```python
from build123d import *

# Parameters (mm, degrees)
BOSS_EXTRUDE1_DEPTH = 5
CUT_EXTRUDE1_DEPTH  = 43.772012023
FILLET1_R           = 2.54
SKETCH3_W           = 20
SKETCH3_H           = 10
BOSS_EXTRUDE2_DEPTH = 48
SKETCH4_W           = 16
SKETCH4_H           = 5
CUT_EXTRUDE4_DEPTH  = 32
FILLET2_R           = 2


with BuildPart() as part:
    # Sketch1 → Boss-Extrude1 (new body)
    with BuildSketch(Plane(origin=(0, 0, 0), x_dir=(1, 0, 0), z_dir=(0, 1, 0))):
        Polygon((-29.999623956, -29.926382831), (30.000376044, -29.926382831), (30.000376044, -9.926382831), (10.000376044, -9.926382831), (10.000376044, 10.073617169), (30.000376044, 10.073617169), (30.000376044, 30.073617169), (-29.999623956, 30.073617169), (-29.999623956, 10.073617169), (-9.999623956, 10.073617169), (-9.999623956, -9.926382831), (-29.999623956, -9.926382831), align=None)
    extrude(amount=BOSS_EXTRUDE1_DEPTH)

    # Sketch2 → Cut-Extrude1 (cut, through all)
    with BuildSketch(Plane(origin=(0, 5, 0), x_dir=(1, 0, 0), z_dir=(0, 1, 0))):
        with BuildLine():
            Line((-18.549247911, 18.573617169), (18.55, 18.573617169))
            ThreePointArc((18.55, 18.573617169), (19.575304833, 18.998312337), (20, 20.023617169))
            Line((20, 20.023617169), (20, 20.123617169))
            ThreePointArc((20, 20.123617169), (19.575304833, 21.148922002), (18.55, 21.573617169))
            Line((18.55, 21.573617169), (-18.549247911, 21.573617169))
            ThreePointArc((-18.549247911, 21.573617169), (-19.574552744, 21.148922002), (-19.999247911, 20.123617169))
            Line((-19.999247911, 20.123617169), (-19.999247911, 20.023617169))
            ThreePointArc((-19.999247911, 20.023617169), (-19.574552744, 18.998312337), (-18.549247911, 18.573617169))
        make_face()
        with BuildLine():
            Line((-18.549623956, -21.426382831), (18.550376044, -21.426382831))
            ThreePointArc((18.550376044, -21.426382831), (19.575680877, -21.001687663), (20.000376044, -19.976382831))
            Line((20.000376044, -19.976382831), (20.000376044, -19.876382831))
            ThreePointArc((20.000376044, -19.876382831), (19.575680877, -18.851077998), (18.550376044, -18.426382831))
            Line((18.550376044, -18.426382831), (-18.549623956, -18.426382831))
            ThreePointArc((-18.549623956, -18.426382831), (-19.574928788, -18.851077998), (-19.999623956, -19.876382831))
            Line((-19.999623956, -19.876382831), (-19.999623956, -19.976382831))
            ThreePointArc((-19.999623956, -19.976382831), (-19.574928788, -21.001687663), (-18.549623956, -21.426382831))
        make_face()
    extrude(amount=-CUT_EXTRUDE1_DEPTH, mode=Mode.SUBTRACT)

    # Fillet1
    fillet1_edges = [part.edges().sort_by_distance(p)[0] for p in [
        (-29.999623956, 2.5, -10.073617169),
        (-29.999623956, 2.5, -30.073617169),
        (30.000376044, 2.5, -30.073617169),
        (30.000376044, 2.5, -10.073617169),
        (10.000376044, 2.5, -10.073617169),
        (10.000376044, 2.5, 9.926382831),
        (30.000376044, 2.5, 9.926382831),
        (30.000376044, 2.5, 29.926382831),
        (-29.999623956, 2.5, 29.926382831),
        (-29.999623956, 2.5, 9.926382831),
        (-9.999623956, 2.5, 9.926382831),
        (-9.999623956, 2.5, -10.073617169),
    ]]
    fillet(fillet1_edges, radius=FILLET1_R)

    # Sketch3 → Boss-Extrude2 (add)
    with BuildSketch(Plane(origin=(0, 5, 0), x_dir=(1, 0, 0), z_dir=(0, 1, 0))):
        Rectangle(SKETCH3_W, SKETCH3_H)
    extrude(amount=BOSS_EXTRUDE2_DEPTH)

    # Sketch4 → Cut-Extrude4 (cut)
    with BuildSketch(Plane(origin=(0, 0, -5), x_dir=(-1, 0, 0), z_dir=(0, 0, -1))):
        with Locations((0, 38.5)):
            Rectangle(SKETCH4_W, SKETCH4_H)
    extrude(amount=-CUT_EXTRUDE4_DEPTH, mode=Mode.SUBTRACT)

    # Fillet2
    fillet2_edges = [part.edges().sort_by_distance(p)[0] for p in [
        (0.000188022, 5, 5),
        (0.000188022, 5, -5),
        (10, 53, 0),
        (-10, 53, 0),
        (-8, 41, 0),
        (-8, 36, 0),
        (8, 36, 0),
        (8, 41, 0),
    ]]
    fillet(fillet2_edges, radius=FILLET2_R)


solid = part.part
```
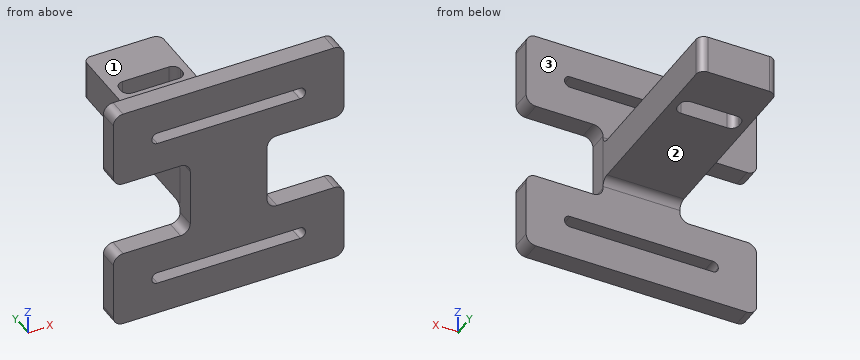
CAD build for the part. Positions are in the model's coordinates, mm. Face numbers are marked on the shaded views. A direction names the side the tool comes from. Round coordinates to 2 decimals unless told otherwise and drop trailing zeros. Order: outer loops, then holes, each group sorted by start corner. A loop starts at its lowest first (then second) coordinate and runs counter-clockwise, first axis right, second up.
Item 1: Saw through at B-B on y = 37. Write the cut outline in (x, z), then the cut area to 3 significant figures.
Item 2: Saw through at A-A on x = -16. Write the cut outline in (y, z), then the cut area to 3 significant figures.
Item 3: Saw through at D-D on x = -22. Write the cut outline in (y, z).
Item 4: Pin check, flat tips, straight feed: pin 1 (3 mm diameter, centred on x = -1, z = -1.5, fed in from -Y); pin 2 (2 mm diameter, centred on x = 8, z = 20.5, fed in from +Y); pin 3 (7 mm diameter, centred on y = 38.5, z = -1.5, fed in from +X); pin 4 (6 mm diameter, centred on x = 3.5, y = 22, fed in from -Z). Stop position of each tip, or through.
Item 5: Probe line 1 along Y through (x, z) = (2, 0); line 2 along Z through (x, y) = (-7.5, 15.5); line 3 along Y through (x, z) = (26, 24). List the from-to ranges inside material, lowest first.
Item 6: Tool access for the marked faces 1, 2 and 3: list every direction of +Z, -Z, +X, -X, +Y, -Y with a clear straight run to the whole face (end or side of a thin tool).
Reported:
1. outline: (-10, -5) - (-7.73, -5) - (-7.73, 5) - (-10, 5) - close; (7.73, -5) - (10, -5) - (10, 5) - (7.73, 5) - close
1. area: 45.4 mm2
2. outline: (0, -30.07) - (5, -30.07) - (5, -21.57) - (0, -21.57) - close; (0, -18.57) - (5, -18.57) - (5, -10.07) - (0, -10.07) - close; (0, 9.93) - (5, 9.93) - (5, 18.43) - (0, 18.43) - close; (0, 21.43) - (5, 21.43) - (5, 29.93) - (0, 29.93) - close
2. area: 170 mm2
3. outline: (0, -30.07) - (5, -30.07) - (5, -10.07) - (0, -10.07) - close; (0, 9.93) - (5, 9.93) - (5, 29.93) - (0, 29.93) - close
4. pin 1: stops at y = 0
4. pin 2: stops at y = 5
4. pin 3: stops at x = 10
4. pin 4: stops at z = -5
5. line 1: y = 0 to 36, 41 to 53
5. line 2: z = -5 to 5
5. line 3: y = 0 to 5
6. face 1: +Z, +X, -X, +Y
6. face 2: -Z, +X, -X, +Y
6. face 3: +X, -X, +Y
